For this review, take the finished solid that the model builds, in its own axes (mm). A direction names the side the tool comes from. Give positions to 0.01 mm unless a question says otherwise; leave off trailing zeros. Order: outer loops, then holes, each group sorted by start corner. A loop starts at its lowest first (then second) coordinate and runs counter-clockwise, first axis right, second up. Notation, with made-up numbers: (3.25, 43.25) -> (10.25, 43.25) arc R20 ccw to (10.25, 52.25) -> close; hole circle Ø10 at (70.5, 48). An arc over 180 degrees is marked (long way). One line per item, written item: value. Start each with the question number.
from build123d import *

# Parameters (mm, degrees)
F0_R      = 5.2
F0_R_2    = 2
F1_DEPTH  = 1.5
F2_R      = 5.2
F3_DEPTH  = 12.5
F4_R      = 5.2
F4_R_2    = 2
F5_DEPTH  = 13
F6_R      = 5.2
F7_DEPTH  = 6
F8_R      = 4
F9_R      = 1.5
F10_DEPTH = 12.5


with BuildPart() as f1:
    # F0 (on Top) → F1 (new body)
    with BuildSketch(Plane.XY):
        Circle(F0_R)
        Circle(F0_R_2, mode=Mode.SUBTRACT)
    extrude(amount=F1_DEPTH)

    # F2 (on face) → F3 (join)
    with BuildSketch(Plane.XY.offset(1.5)):
        Circle(F2_R)
        Polygon((0, 3.9259818305), (3.4, 1.9629909152), (3.4, -1.9629909152), (0, -3.9259818305), (-3.4, -1.9629909152), (-3.4, 1.9629909152), align=None, mode=Mode.SUBTRACT)
    extrude(amount=F3_DEPTH)

    # F4 (on face) → F5 (join)
    with BuildSketch(Plane.XY.offset(14)):
        Circle(F4_R)
        Polygon((-3.4, -1.9629909152), (-3.4, 1.9629909152), (0, 3.9259818305), (3.4, 1.9629909152), (3.4, -1.9629909152), (0, -3.9259818305), align=None, mode=Mode.SUBTRACT)
        Polygon((0, 3.9259818305), (-3.4, 1.9629909152), (-3.4, -1.9629909152), (0, -3.9259818305), (3.4, -1.9629909152), (3.4, 1.9629909152), align=None)
        Circle(F4_R_2, mode=Mode.SUBTRACT)
    extrude(amount=F5_DEPTH)

    # F6 (on face) → F7 (join)
    with BuildSketch(Plane.XY.offset(27)):
        Circle(F6_R)
    extrude(amount=F7_DEPTH)

    # F8
    f8_edges = [f1.edges().sort_by_distance(p)[0] for p in [
        (-5.2, 0, 33),
    ]]
    fillet(f8_edges, radius=F8_R)

    # F9 (on Front) → F10 (cut, symmetric)
    with BuildSketch(Plane.XZ):
        with Locations((0, 28)):
            Circle(F9_R)
    extrude(amount=F10_DEPTH, both=True, mode=Mode.SUBTRACT)


solid = f1.part
Q1. For faces 1 (the cylindrical face through (-0.195, -0.073, 29.487)), 2 (the cylindrical face through (0, -2, 1)), 3 (the flat face through (-1.724, 2.931, 7.662)), list the 3-axis set-ups (+Z, -Z, +X, -X, +Y, -Y) from which the entire face can be reached by the end or side of a thin tool; tool diameter is ignored.
Q2. Mouldability with a two-part tool opening along Y and no side actions: class faces 4 (the cylindrical face through (4.96, 1.56, 14.3)), 5 (the flat face through (2.2, 0.1, 0)), 6 (the flat face through (-1.676, -2.958, 7.662)), 7 (the flat face through (3.4, 0, 8)) as pulls with the +Y half, pulls with the -Y half, needs draft (parallel to the pull), parting line crosses it, or undercut.
Q3. For line 1 along Y through (x, z) = (0, 18.5); line 2 along X through (y, z) = (-0.25, 11); line 3 along Y through (x, z) = (-0.25, 10.5), list the stretches that pass through material, from the lowest coordinate up.
Q4. For pin 1 Ø1.2 at (y, z) = (-1, 6) entering from +X; pin 2 Ø1 at (y, z) = (2, 9.5) entering from +X; pin 3 Ø1.5 at (x, y) = (0.5, -3.5) entering from +Z, all flat-tipped, find the tip position at first contact; note any pin that passes through.
Q5. Take a section at D-D (z = 14.5). State the section outline as (x, y) points.
Q6. Take a section at B-B (z = 28). State the section outline as (x, y) points.
Q7. Take a section at A-A (z = 7). State the section outline as (x, y) points, and give its area (3 significant figures).
Q8. Take a section at C-C (y = -3.5). State how many separate pieces and enclosed holes the cut face has, and give its area (3 significant figures).
Answers below:
1. face 1: +Y, -Y
1. face 2: -Z
1. face 3: none
2. face 4: parting line crosses it
2. face 5: needs draft
2. face 6: undercut
2. face 7: undercut
3. line 1: y = -5.2 to -2, 2 to 5.2
3. line 2: x = -5.19 to -3.4, 3.4 to 5.19
3. line 3: y = -5.19 to -3.78, 3.78 to 5.19
4. pin 1: stops at x = 5.18
4. pin 2: stops at x = 4.98
4. pin 3: stops at z = 32.67
5. outline: circle Ø10.4 at (0, 0); hole circle Ø4 at (0, 0)
6. outline: (-1.5, -4.98) -> (-1.5, 4.98) arc R5.2 ccw to start; (1.5, -4.98) arc R5.2 ccw to (1.5, 4.98) -> close
7. outline: circle Ø10.4 at (0, 0); hole (-3.4, -1.96) -> (0, -3.93) -> (3.4, -1.96) -> (3.4, 1.96) -> (0, 3.93) -> (-3.4, 1.96) -> close
7. area: 44.9 mm²
8. separate pieces: 1
8. enclosed holes: 2
8. area: 217 mm²
